from build123d import *

# Parameters (mm, degrees)
SKETCH1_R           = 1.25
BOSS_EXTRUDE1_DEPTH = 5
FILLET1_R           = 5


with BuildPart() as part:
    # Sketch1 → Boss-Extrude1 (new body)
    with BuildSketch(Plane.XY):
        Polygon((-38, 74.828427125), (0, 112.828427125), (38, 74.828427125), (38, 104.828427125), (0, 142.828427125), (-38, 104.828427125), align=None)
        with Locations((-31.819805153, 96.008621971)):
            Circle(SKETCH1_R, mode=Mode.SUBTRACT)
        with Locations((-21.213203436, 106.615223689)):
            Circle(SKETCH1_R, mode=Mode.SUBTRACT)
        with Locations((-10.606601718, 117.221825407)):
            Circle(SKETCH1_R, mode=Mode.SUBTRACT)
        with Locations((0, 127.828427125)):
            Circle(SKETCH1_R, mode=Mode.SUBTRACT)
        with Locations(Location((10.606601718, 117.221825407, 0), (0, 0, 180))):
            Circle(SKETCH1_R, mode=Mode.SUBTRACT)
        with Locations(Location((21.213203436, 106.615223689, 0), (0, 0, 180))):
            Circle(SKETCH1_R, mode=Mode.SUBTRACT)
        with Locations(Location((31.819805153, 96.008621971, 0), (0, 0, 180))):
            Circle(SKETCH1_R, mode=Mode.SUBTRACT)
    extrude(amount=BOSS_EXTRUDE1_DEPTH)

    # Fillet1
    fillet1_edges = [part.edges().sort_by_distance(p)[0] for p in [
        (-38, 104.828427125, 2.5),
        (0, 142.828427125, 2.5),
        (38, 104.828427125, 2.5),
        (38, 74.828427125, 2.5),
        (0, 112.828427125, 2.5),
        (-38, 74.828427125, 2.5),
    ]]
    fillet(fillet1_edges, radius=FILLET1_R)


solid = part.part
Geometry: final body of the model. Coordinates: model frame, mm. A direction names the side the tool comes from. Round coordinates to 2 decimals unless told otherwise and drop trailing zeros. Order: outer loops, then holes, each group sorted by start corner. A loop starts at its lowest first (then second) coordinate and runs counter-clockwise, first axis right, second up. Notation, with made-up numbers: (74.5, 35.5) - (87.5, 35.5) arc R28 ccw to (87.5, 66.5) - close; hole circle Ø7 at (26.5, 43.25). An arc over 180 degrees is marked (long way). Write each question's results on one line, items separated by ' | '.
Item 1: Section B-B, the plane z = 4. Return the cut outline in (x, y), and give its area (3 significant figures).
Completed:
outline: (-38, 86.9) arc R5 ccw to (-29.46, 83.36) - (-3.54, 109.29) arc R5 cw to (3.54, 109.29) - (29.46, 83.36) arc R5 ccw to (38, 86.9) - (38, 102.76) arc R5 ccw to (36.54, 106.29) - (3.54, 139.29) arc R5 ccw to (-3.54, 139.29) - (-36.54, 106.29) arc R5 ccw to (-38, 102.76) - close; hole circle Ø2.5 at (-31.82, 96.01); hole circle Ø2.5 at (-21.21, 106.62); hole circle Ø2.5 at (-10.61, 117.22); hole circle Ø2.5 at (0, 127.83); hole circle Ø2.5 at (10.61, 117.22); hole circle Ø2.5 at (21.21, 106.62); hole circle Ø2.5 at (31.82, 96.01) | area: 2,180 mm^2
Item 2: Section D-D, the plane x = 13. Return the cut outline in (y, z), and give its area (3 significant figures).
Completed:
outline: (99.83, 0) - (129.83, 0) - (129.83, 5) - (99.83, 5) - close | area: 150 mm^2
Item 3: Reachability of faces 1 (the flat face through (-19.805, 123.024, 2.465)), 2 (the flat face through (-16.68, 96.15, 2.46)) from +Z, -Z, +X, -X, +Y, -Y: full face, straight path, thin tool, end or side. Return the list, or none.
Completed:
face 1: +Z, -Z, -X, +Y | face 2: +Z, -Z, -Y
Item 4: Material intervals for line 1 along Y through (x, z) = (0, 1.65); line 2 along X through (y, z) = (107, 1.25); line 3 along Y through (x, z) = (32.5, 3.7), sorted ascending. Write a range as [from, to].
Completed:
line 1: [110.76, 126.58], [129.08, 140.76] | line 2: [-35.83, -22.4], [-20.02, -5.83], [5.83, 20.02], [22.4, 35.83] | line 3: [81.92, 94.96], [97.06, 110.33]
Item 5: Section A-A, the plane x = 0. Return the cut outline in (y, z), and give its area (4 significant figures).
Completed:
outline: (110.76, 0) - (126.58, 0) - (126.58, 5) - (110.76, 5) - close; (129.08, 0) - (140.76, 0) - (140.76, 5) - (129.08, 5) - close | area: 137.5 mm^2
Item 6: Mould query, pull axis Y, two halves, no side actions, for faces 3 (the flat face through (16.32, 96.51, 2.46)), 4 (the cylindrical face through (10.769, 115.982, 2.465)), 5 (the cylindrical face through (31.148, 94.955, 2.465)), 6 (the cylindrical face through (37.63, 104.65, 2.54)). Classes: pulls with the +Y half, pulls with the -Y half, needs draft (parallel to the pull), parting line crosses it, or undercut.
Completed:
face 3: pulls with the -Y half | face 4: undercut | face 5: undercut | face 6: pulls with the +Y half
Item 7: Section C-C, the plane y = 92.5. Return the cut outline in (x, z).
Completed:
outline: (-38, 0) - (-20.33, 0) - (-20.33, 5) - (-38, 5) - close; (20.33, 0) - (38, 0) - (38, 5) - (20.33, 5) - close
Item 8: First-contact query: pin 1 Ø3 at (x, y) = (0, 127.83) entering from +Z. Flat tip, straight axial feed; report the tip coordinate or a pass-through.
Completed:
pin 1: z = 5
